Geometry: final body of the model. Coordinates: model frame, mm. Give positions to 0.01 mm unless a question says otherwise; leave off trailing zeros. Order: outer loops, then holes, each group sorted by start corner. A loop starts at its lowest first (then second) coordinate and runs counter-clockwise, first axis right, second up. Notation, with made-up numbers: (-12.5, 14.25) -> (42.5, 14.25) arc R29 cw to (42.5, 39.25) -> close; hole circle Ø1 at (-30.75, 76). An arc over 180 degrees is marked (long way). Answer in a Markdown table with one row per item. Add a question column.
Q1. Cut plane C-C on x = -6.25. Return the cut outline in (y, z), and give its area (4 significant figures).
Q2. Contact query for flat-ended pins moving along their axis: P1, Ø1, axis at y = -1, z = 117.5, coming from the +X side; P2, Ø4, axis at x = -5, z = 47, coming from the -Y side; P3, Ø0.6, axis at y = -3.5, z = 116.5, coming from the -X side. Output: stop coordinate, or through.
Q3. Cut plane A-A on z = 12. Return the cut outline in (x, y), and give its area (3 significant figures).
Q4. Cut plane B-B on z = 50. Return the cut outline in (x, y).
Q5. Line query: line 1 along Y through (x, z) = (0, 10.75); line 2 along Z through (x, y) = (4, -3.5); line 3 along Y through (x, z) = (2.25, 6.5). Output: solid intervals per line, ascending. Write a range as from..to.
Q6. Cut plane D-D on x = 6.5. Return the cut outline in (y, z), and give its area (3 significant figures).
from build123d import *

# Parameters (mm, degrees)
SKETCH_1_R             = 5
EXTRUDE_1_DEPTH        = 114
SKETCH_2_R             = 8
EXTRUDE_2_DEPTH        = 4
SKETCH_4_W             = 1.5
SKETCH_4_H             = 19.56005024
CUT_EXTRUDE_1_DEPTH    = 2
HOLE_WIZARD_M8_1_D     = 6.8
HOLE_WIZARD_M8_1_DEPTH = 15
HOLE_WIZARD_M8_1_TIP   = 2.042926105


with BuildPart() as part:
    # 草图1 → 凸台-拉伸1 (new body)
    with BuildSketch(Plane.XY):
        with Locations(Location((0, 0, 0), (0, 0, 180))):
            Circle(SKETCH_1_R)
    extrude(amount=EXTRUDE_1_DEPTH)

    # 草图2 → 凸台-拉伸2 (add)
    with BuildSketch(Plane.XY.offset(114)):
        Circle(SKETCH_2_R)
    extrude(amount=EXTRUDE_2_DEPTH)

    # 草图4 → 切除-拉伸1 (cut)
    with BuildSketch(Plane.XY.offset(118)):
        Rectangle(SKETCH_4_W, SKETCH_4_H)
    extrude(amount=-CUT_EXTRUDE_1_DEPTH, mode=Mode.SUBTRACT)

    # M8 螺纹孔的螺纹孔钻头1
    with Locations(Plane(origin=(0, 0, 0), x_dir=(-1, 0, 0), z_dir=(0, 0, -1))):
        with Locations((0, 0)):
            Hole(HOLE_WIZARD_M8_1_D / 2, depth=HOLE_WIZARD_M8_1_DEPTH)
            with Locations((0, 0, -(HOLE_WIZARD_M8_1_DEPTH + HOLE_WIZARD_M8_1_TIP / 2))):  # 118° drill point
                Cone(0, HOLE_WIZARD_M8_1_D / 2, HOLE_WIZARD_M8_1_TIP, mode=Mode.SUBTRACT)


solid = part.part
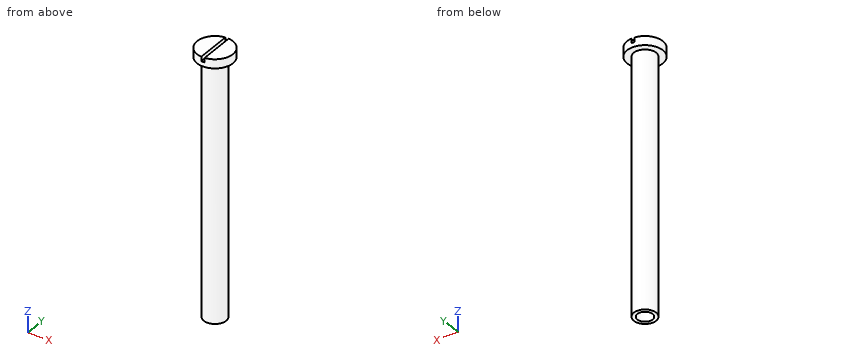
Completed:
| question | item | result |
|---|---|---|
| 1 | outline | (-4.99, 114) -> (4.99, 114) -> (4.99, 118) -> (-4.99, 118) -> close |
| 1 | area | 39.95 mm² |
| 2 | P1 | stops at x = 7.98 |
| 2 | P2 | stops at y = -4 |
| 2 | P3 | stops at x = -7.33 |
| 3 | outline | circle Ø10 at (0, 0); hole circle Ø6.8 at (0, 0) |
| 3 | area | 42.2 mm² |
| 4 | outline | circle Ø10 at (0, 0) |
| 5 | line 1 | y = -5..-3.4, 3.4..5 |
| 5 | line 2 | z = 114..118 |
| 5 | line 3 | y = -4.47..-2.55, 2.55..4.47 |
| 6 | outline | (-4.66, 114) -> (4.66, 114) -> (4.66, 118) -> (-4.66, 118) -> close |
| 6 | area | 37.3 mm² |
